from build123d import *

# Parameters (mm, degrees)
SKETCH1_W           = 21
SKETCH1_H           = 13
SKETCH1_R           = 1.4732
BOSS_EXTRUDE1_DEPTH = 6.35
SKETCH2_R           = 3.175
CUT_EXTRUDE1_DEPTH  = 13


with BuildPart() as part:
    # Sketch1 → Boss-Extrude1 (new body)
    with BuildSketch(Plane(origin=(0, 0, 0), x_dir=(1, 0, 0), z_dir=(0, 1, 0))):
        with Locations((20.5, -6.5)):
            Rectangle(SKETCH1_W, SKETCH1_H)
        with Locations(Location((14.15, -6.5, 0), (0, 0, 270))):
            Circle(SKETCH1_R, mode=Mode.SUBTRACT)
        with Locations(Location((26.85, -6.5, 0), (0, 0, 270))):
            Circle(SKETCH1_R, mode=Mode.SUBTRACT)
    extrude(amount=BOSS_EXTRUDE1_DEPTH)

    # Sketch2 → Cut-Extrude1 (cut)
    with BuildSketch(Plane(origin=(0, 0, 0), x_dir=(-1, 0, 0), z_dir=(0, 0, -1))):
        with Locations((-20.5, 0)):
            Circle(SKETCH2_R)
    extrude(amount=-CUT_EXTRUDE1_DEPTH, mode=Mode.SUBTRACT)


solid = part.part
Work out the finished part from the listing and answer in its coordinate system (mm). Give positions to 0.01 mm unless a question says otherwise; leave off trailing zeros. Loops run counter-clockwise (first coordinate to the right, second up) from the corner with the lowest first, then second, coordinate; pieces in that order, holes last. Notation, with made-up numbers: (46.5, -14) -> (103.5, -14) arc R7 cw to (103.5, -4) -> close; hole circle Ø6 at (-3.75, 56). An arc over 180 degrees is marked (long way). Use a Markdown table: item, result. Add a question column.
1. Determine the mould class of faces 1 (the cylindrical face through (13.254, 3.131, 5.331)), 2 (the flat face through (20, 4, 13)), 3 (the cylindrical face through (25.41, 3.13, 6.18)), 4 (the cylindrical face through (20.43, 3.174, 6.409)) for opening direction Z: released by +Z, released by -Z, zero draft, split by the parting line, or undercut.
2. Section A-A on z = 6.5 is taken. Determine the outline of the cut face in (x, y) (3 decimals), and give its area (3 significant figures).
3. A flat-ended cylindrical pin translates along its axis: pin 1 Ø1.8 at (x, z) = (26.85, 6.5) entering from +Y. Find the tip coordinate at first contact, or state that the pin passes through.
4. Section B-B on y = 2.5 is taken. Determine the outline of the cut face in (x, z).
5. Section C-C on x = 26.85 is taken. Determine the outline of the cut face in (y, z).
6. Section D-D on y = 3.5 is taken. Determine the outline of the cut face in (x, z).
7. Find the intervals of material crossed by probe 1 along X at (y, z) = (3.75, 6.5); probe 2 along X at (y, z) = (2.25, 7.25); probe 3 along X at (y, z) = (1.5, 6.5), in increasing order.
Results below:
| question | item | result |
|---|---|---|
| 1 | face 1 | undercut |
| 1 | face 2 | released by +Z |
| 1 | face 3 | undercut |
| 1 | face 4 | zero draft |
| 2 | outline | (10, 0) -> (12.677, 0) -> (12.677, 6.35) -> (10, 6.35) -> close; (15.623, 0) -> (17.325, 0) arc R3.175 cw to (23.675, 0) -> (25.377, 0) -> (25.377, 6.35) -> (15.623, 6.35) -> close; (28.323, 0) -> (31, 0) -> (31, 6.35) -> (28.323, 6.35) -> close |
| 2 | area | 80.1 mm^2 |
| 3 | pin 1 | passes through |
| 4 | outline | (10, 0) -> (18.54, 0) -> (18.54, 13) -> (10, 13) -> close; (22.46, 0) -> (31, 0) -> (31, 13) -> (22.46, 13) -> close; hole circle Ø2.95 at (14.15, 6.5); hole circle Ø2.95 at (26.85, 6.5) |
| 5 | outline | (0, 0) -> (6.35, 0) -> (6.35, 5.03) -> (0, 5.03) -> close; (0, 7.97) -> (6.35, 7.97) -> (6.35, 13) -> (0, 13) -> close |
| 6 | outline | (10, 0) -> (31, 0) -> (31, 13) -> (10, 13) -> close; hole circle Ø2.95 at (14.15, 6.5); hole circle Ø2.95 at (26.85, 6.5) |
| 7 | probe 1 | x = 10 to 12.68, 15.62 to 25.38, 28.32 to 31 |
| 7 | probe 2 | x = 10 to 12.88, 15.42 to 18.26, 22.74 to 25.58, 28.12 to 31 |
| 7 | probe 3 | x = 10 to 12.68, 15.62 to 17.7, 23.3 to 25.38, 28.32 to 31 |
